from build123d import *

# Parameters (mm, degrees)
SKETCH1_W           = 42
SKETCH1_H           = 60
BOSS_EXTRUDE1_DEPTH = 10
BOSS_EXTRUDE2_DEPTH = 25
SKETCH3_R           = 4
CUT_EXTRUDE1_DEPTH  = 15
SKETCH4_R           = 2.5
CUT_EXTRUDE2_DEPTH  = 15


with BuildPart() as part:
    # Sketch1 → Boss-Extrude1 (new body)
    with BuildSketch(Plane(origin=(0, 0, 0), x_dir=(1, 0, 0), z_dir=(0, 1, 0))):
        with Locations((21, 30)):
            Rectangle(SKETCH1_W, SKETCH1_H)
    extrude(amount=BOSS_EXTRUDE1_DEPTH)

    # Sketch2 → Boss-Extrude2 (add)
    with BuildSketch(Plane(origin=(0, 10, 0), x_dir=(1, 0, 0), z_dir=(0, 1, 0))):
        with BuildLine():
            Line((0, 20), (21, 20))
            ThreePointArc((21, 20), (31, 30), (21, 40))
            Line((21, 40), (0, 40))
            Line((0, 40), (0, 60))
            Line((0, 60), (42, 60))
            Line((42, 60), (42, 0))
            Line((42, 0), (0, 0))
            Line((0, 0), (0, 20))
        make_face()
    extrude(amount=BOSS_EXTRUDE2_DEPTH)

    # Sketch3 → Cut-Extrude1 (cut)
    with BuildSketch(Plane.ZY):
        with Locations((-10, 22.5)):
            Circle(SKETCH3_R)
        with Locations(Location((-50, 22.5, 0), (0, 0, 180))):
            Circle(SKETCH3_R)
    extrude(amount=-CUT_EXTRUDE1_DEPTH, mode=Mode.SUBTRACT)

    # Sketch4 → Cut-Extrude2 (cut)
    with BuildSketch(Plane(origin=(0, 10, 0), x_dir=(1, 0, 0), z_dir=(0, 1, 0))):
        with Locations(Location((20.85, 30, 0), (0, 0, 270))):
            Circle(SKETCH4_R)
    extrude(amount=-CUT_EXTRUDE2_DEPTH, mode=Mode.SUBTRACT)


solid = part.part
Part model, mm, in its own coordinate system. A direction names the side the tool comes from. Give positions to 0.01 mm unless a question says otherwise; leave off trailing zeros. Loops run counter-clockwise (first coordinate to the right, second up) from the corner with the lowest first, then second, coordinate; pieces in that order, holes last. Notation, with made-up numbers: M 58.25,88 L 79.25,88 A16 ccw 79.25,100 Z; hole C -34.5,-35.5 d9. An arc over 180 degrees is marked long. Put each result on its own line as item: value. Start each with the question number.
1) Saw through at B-B (x = 12.5). List the corners of the cut face in (y, z).
2) Saw through at C-C (y = 30). List the corners of the cut face in (x, z).
3) Saw through at A-A (z = -30). List the corners of the cut face in (x, y), then the cut area to 3 significant figures.
4) Pull direction Z, two halves, no side cores. Call faces 1 (the flat face through (15, 10, -30)), 2 (the flat face through (21, 17, -60)), 3 (the flat face through (31, 35, -24)), 4 (the flat face through (21, 17, 0)): +Z half, -Z half, draft (parallel to the pull), parting line (faces both ways), or undercut.
5) 3-axis set-ups, long thin cutter, end or side, ignore diameter. For faces 5 (the flat face through (15, 23, -10)), 6 (the cylindrical face through (31, 22, -30)), 7 (the flat face through (0, 9, -30)): which of +Z, -Z, +X, -X, +Y, -Y reach the whole face in a straight line?
6) Probe probe 1 along Z at (x, y) = (17.5, 12); probe 2 along Y at (x, z) = (8.5, -50); probe 3 along Z at (x, y) = (7, 26). List the from-to ranges inside material, lowest first.
7) Flat gauge pins, fed straight in: pin 1 (4 mm diameter, centred on x = 20.85, z = -30, fed in from +Y); pin 2 (2.5 mm diameter, centred on y = 23.5, z = -9, fed in from -X). Where does each tip first touch, or does it go through?
8) Saw through at D-D (z = -10). List the corners of the cut face in (x, y).
Numbers:
1. outline: M 0,-60 L 35,-60 L 35,-40 L 10,-40 L 10,-20 L 35,-20 L 35,0 L 0,0 Z; hole C 22.5,-50 d8; hole C 22.5,-10 d8
2. outline: M 0,-60 L 42,-60 L 42,0 L 0,0 L 0,-20 L 21,-20 A10 cw 21,-40 L 0,-40 Z
3. outline: M 0,0 L 18.35,0 L 18.35,10 L 0,10 Z; M 23.35,0 L 42,0 L 42,35 L 31,35 L 31,10 L 23.35,10 Z
3. area: 645 mm^2
4. face 1: undercut
4. face 2: -Z half
4. face 3: draft
4. face 4: +Z half
5. face 5: -X
5. face 6: -X, +Y
5. face 7: +Z, -Z, -X, +Y, -Y
6. probe 1: -60 to -40, -20 to 0
6. probe 2: 0 to 18.5, 26.5 to 35
6. probe 3: -60 to -51.94, -48.06 to -40, -20 to -11.94, -8.06 to 0
7. pin 1: through
7. pin 2: x = 15
8. outline: M 0,0 L 42,0 L 42,35 L 0,35 L 0,26.5 L 15,26.5 L 15,18.5 L 0,18.5 Z
